Here's how the part is built. I have some questions about the finished solid (model axes, mm). Face numbers are marked on the shaded views. Round coordinates to 2 decimals unless told otherwise and drop trailing zeros. Loops run counter-clockwise (first coordinate to the right, second up) from the corner with the lowest first, then second, coordinate; pieces in that order, holes last. Notation, with made-up numbers: M -19,7 L 13,7 A23 cw 13,22 Z; hole C 18,-40 d8. An arc over 180 degrees is marked long. Use a Markdown table: item, result.
from build123d import *

# Parameters (mm, degrees)
CYLINDER005_R     = 1.58
CYLINDER005_DEPTH = 20
CYLINDER001_R     = 2
CYLINDER001_DEPTH = 20
CYLINDER002_R     = 1.58
CYLINDER002_DEPTH = 20
CYLINDER003_R     = 1.58
CYLINDER003_DEPTH = 20
CYLINDER004_R     = 1.58
CYLINDER004_DEPTH = 20
CYLINDER_R        = 19
CYLINDER_DEPTH    = 19
BOX_W             = 40
BOX_H             = 40
BOX_DEPTH         = 20


with BuildPart() as cylinder005:
    # Cylinder005 → Cylinder005 (new body)
    with BuildSketch(Plane(origin=(4.95, 4.6, -2), x_dir=(1, 0, 0), z_dir=(0, 0, 1))):
        Circle(CYLINDER005_R)
    extrude(amount=CYLINDER005_DEPTH)


with BuildPart() as cylinder001:
    # Cylinder001 → Cylinder001 (new body)
    with BuildSketch(Plane.XY.offset(-2)):
        Circle(CYLINDER001_R)
    extrude(amount=CYLINDER001_DEPTH)


with BuildPart() as cylinder002:
    # Cylinder002 → Cylinder002 (new body)
    with BuildSketch(Plane(origin=(-4.95, 4.6, -2), x_dir=(1, 0, 0), z_dir=(0, 0, 1))):
        Circle(CYLINDER002_R)
    extrude(amount=CYLINDER002_DEPTH)


with BuildPart() as cylinder003:
    # Cylinder003 → Cylinder003 (new body)
    with BuildSketch(Plane(origin=(4.95, -4.6, -2), x_dir=(1, 0, 0), z_dir=(0, 0, 1))):
        Circle(CYLINDER003_R)
    extrude(amount=CYLINDER003_DEPTH)


with BuildPart() as cylinder004:
    # Cylinder004 → Cylinder004 (new body)
    with BuildSketch(Plane(origin=(-4.95, -4.6, -2), x_dir=(1, 0, 0), z_dir=(0, 0, 1))):
        Circle(CYLINDER004_R)
    extrude(amount=CYLINDER004_DEPTH)


with BuildPart() as cylinder:
    # Cylinder → Cylinder (new body)
    with BuildSketch(Plane.XY):
        Circle(CYLINDER_R)
    extrude(amount=CYLINDER_DEPTH)


with BuildPart() as cut005:
    # Box → Box (new body)
    with BuildSketch(Plane(origin=(-20, -20, -2), x_dir=(1, 0, 0), z_dir=(0, 0, 1))):
        with Locations((20, 20)):
            Rectangle(BOX_W, BOX_H)
    extrude(amount=BOX_DEPTH)

    # Cut: cut Cylinder
    add(cylinder.part, mode=Mode.SUBTRACT)

    # Cut001: cut Cylinder004
    add(cylinder004.part, mode=Mode.SUBTRACT)

    # Cut002: cut Cylinder003
    add(cylinder003.part, mode=Mode.SUBTRACT)

    # Cut003: cut Cylinder002
    add(cylinder002.part, mode=Mode.SUBTRACT)

    # Cut004: cut Cylinder001
    add(cylinder001.part, mode=Mode.SUBTRACT)

    # Cut005: cut Cylinder005
    add(cylinder005.part, mode=Mode.SUBTRACT)


solid = cut005.part
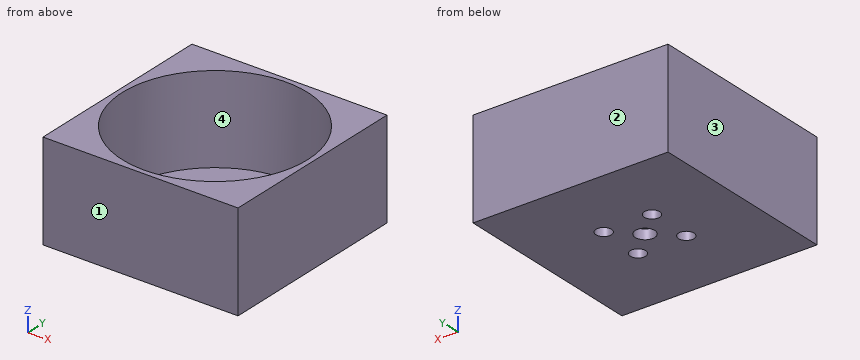
1. Imagine slicing it at C-C, the plane z = 3. Write out the boundary of the cut face in (x, y).
Answer sheet:
| item | result |
|---|---|
| outline | M -20,-20 L 20,-20 L 20,20 L -20,20 Z; hole C 0,0 d38 |
2. Imagine slicing it at D-D, the plane x = -14. Write out the boundary of the cut face in (y, z).
Answer sheet:
| item | result |
|---|---|
| outline | M -20,-2 L 20,-2 L 20,18 L 12.85,18 L 12.85,0 L -12.85,0 L -12.85,18 L -20,18 Z |
3. For pin 1 Ø3.5 at (x, y) = (0, 0) entering from +Z; pin 2 Ø5 at (x, y) = (-2, 15.5) entering from +Z, each with a flat end and sliding along its axis, tell me the tip position at first contact or that it passes through.
Answer sheet:
| item | result |
|---|---|
| pin 1 | through |
| pin 2 | z = 0 |
4. I need wall thicknesses on probe 1 along Y at (x, z) = (-4.95, -1.2); probe 2 along X at (y, z) = (4.6, -0.7); probe 3 along X at (y, z) = (0, -1.6). Which ranges of each line are inside material? Lowest first, please. Write a range as from..to.
Answer sheet:
| item | result |
|---|---|
| probe 1 | -20..-6.18, -3.02..3.02, 6.18..20 |
| probe 2 | -20..-6.53, -3.37..3.37, 6.53..20 |
| probe 3 | -20..-2, 2..20 |
5. We'd pull the mould along Y, two halves only. Please class the marked faces 1, 2, 3 and 4: +Y half, -Y half, draft (parallel to the pull), parting line (faces both ways), or undercut.
Answer sheet:
| item | result |
|---|---|
| face 1 | -Y half |
| face 2 | +Y half |
| face 3 | draft |
| face 4 | undercut |
6. Imagine slicing it at A-A, the plane y = 0. Write out the boundary of the cut face in (x, z).
Answer sheet:
| item | result |
|---|---|
| outline | M -20,-2 L -2,-2 L -2,0 L -19,0 L -19,18 L -20,18 Z; M 2,-2 L 20,-2 L 20,18 L 19,18 L 19,0 L 2,0 Z |
